Can you work these out from the model? Positions are in its coordinate system, mm. Face numbers are marked on the shaded views. A direction names the side the tool comes from. Round coordinates to 2 decimals unless told otherwise and drop trailing zeros. Loops run counter-clockwise (first coordinate to the right, second up) from the corner with the lowest first, then second, coordinate; pieces in that order, holes last.
```python
from build123d import *

# Parameters (mm, degrees)
F0_R     = 60.286911
F0_R_2   = 7.419819
F1_DEPTH = 5
F2_R     = 10.451192
F2_R_2   = 7.419819
F2_R_3   = 5.05785
F2_R_4   = 2.680452
F3_DEPTH = 80


with BuildPart() as f1:
    # F0 (on Top) → F1 (new body)
    with BuildSketch(Plane.XY):
        Circle(F0_R)
        Circle(F0_R_2, mode=Mode.SUBTRACT)
    extrude(amount=F1_DEPTH)

    # F2 (on face) → F3 (join)
    with BuildSketch(Plane.XY.offset(5)):
        Circle(F2_R)
        Circle(F2_R_2, mode=Mode.SUBTRACT)
        with Locations((0, -24.324838)):
            Circle(F2_R_3)
        with Locations((0, -24.324838)):
            Circle(F2_R_4, mode=Mode.SUBTRACT)
        with Locations((-21.065928, -12.162419)):
            Circle(F2_R_3)
        with Locations((-21.065928, -12.162419)):
            Circle(F2_R_4, mode=Mode.SUBTRACT)
        with Locations((0, 24.324838)):
            Circle(F2_R_3)
        with Locations((0, 24.324838)):
            Circle(F2_R_4, mode=Mode.SUBTRACT)
        with Locations((-21.065928, 12.162419)):
            Circle(F2_R_3)
        with Locations((-21.065928, 12.162419)):
            Circle(F2_R_4, mode=Mode.SUBTRACT)
        with Locations((21.065928, 12.162419)):
            Circle(F2_R_3)
        with Locations((21.065928, 12.162419)):
            Circle(F2_R_4, mode=Mode.SUBTRACT)
        with Locations((21.065928, -12.162419)):
            Circle(F2_R_3)
        with Locations((21.065928, -12.162419)):
            Circle(F2_R_4, mode=Mode.SUBTRACT)
    extrude(amount=F3_DEPTH)


solid = f1.part
```
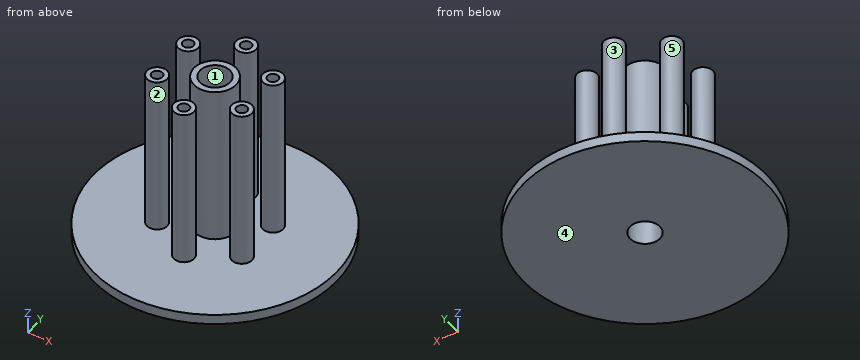
(1) Suppose I cut it at C-C (z = 13). Give the number of separate pieces and of enclosed holes in the cut face, then the cut area to 3 significant figures.
(2) We'd pull the mould along Y, two halves only. Please class the marked faces 3, 4 and 5: released by +Y, released by -Y, zero draft, split by the parting line, or undercut.
(3) If I drill on line 1 (Y direction, x = 0, z = 21); line 2 (X direction, y = -10.5, z = 38.5); line 3 (Y direction, x = -1.5, z = 54.5), over which ranges is the centre line in solid material (lowest first)?
(4) Suppose I cut it at D-D (y = 51.5). Write out the boundary of the cut face in (x, z).
(5) Which directions (+Z, -Z, +X, -X, +Y, -Y) give clear straight access to the entire face, cutting with the end or side of a thin tool? Please do the marked faces 1 and 2.
(6) Suppose I cut it at A-A (x = 0). Write out the boundary of the cut face in (y, z).
(7) Suppose I cut it at B-B (y = 0). Write out the boundary of the cut face in (x, z).
(8) For pin 1 (2.5 mm diameter, centred on x = 20.5, y = 11, fed in from +Z); pin 2 (1 mm diameter, centred on x = -4, z = 75.5, fed in from +Y); pin 3 (12 mm diameter, centred on y = -26.5, z = 69.5, fed in from -X), each with a flat end and sliding along its axis, tell me the tip position at first contact or that it passes through.
Check result:
1. separate pieces: 7
1. enclosed holes: 7
1. area: 517 mm2
2. face 3: undercut
2. face 4: zero draft
2. face 5: undercut
3. line 1: y = -29.38 to -27.01, -21.64 to -19.27, -10.45 to -7.42, 7.42 to 10.45, 19.27 to 21.64, 27.01 to 29.38
3. line 2: x = -25.84 to -23.17, -18.96 to -16.29, 16.29 to 18.96, 23.17 to 25.84
3. line 3: y = -29.16 to -26.55, -22.1 to -19.49, -10.34 to -7.27, 7.27 to 10.34, 19.49 to 22.1, 26.55 to 29.16
4. outline: (-31.34, 0) - (31.34, 0) - (31.34, 5) - (-31.34, 5) - close
5. face 1: +Z, -Z
5. face 2: +Z
6. outline: (-60.29, 0) - (-7.42, 0) - (-7.42, 85) - (-10.45, 85) - (-10.45, 5) - (-19.27, 5) - (-19.27, 85) - (-21.64, 85) - (-21.64, 5) - (-27.01, 5) - (-27.01, 85) - (-29.38, 85) - (-29.38, 5) - (-60.29, 5) - close; (7.42, 0) - (60.29, 0) - (60.29, 5) - (29.38, 5) - (29.38, 85) - (27.01, 85) - (27.01, 5) - (21.64, 5) - (21.64, 85) - (19.27, 85) - (19.27, 5) - (10.45, 5) - (10.45, 85) - (7.42, 85) - close
7. outline: (-60.29, 0) - (-7.42, 0) - (-7.42, 85) - (-10.45, 85) - (-10.45, 5) - (-60.29, 5) - close; (7.42, 0) - (60.29, 0) - (60.29, 5) - (10.45, 5) - (10.45, 85) - (7.42, 85) - close
8. pin 1: stops at z = 5
8. pin 2: stops at y = 27.98
8. pin 3: stops at x = -5.06
